Autodesk Inventor part; units mm, degrees
ref_plane "Work Plane1" through (104.775, 0, 0) normal (0, 0, -1) x (1, 0, 0)
ref_plane "YZ Plane" through (0, 0, 0) normal (1, 0, 0) x (0, 1, 0)
ref_plane "XZ Plane" through (0, 0, 0) normal (0, 1, 0) x (-1, 0, 0)
sketch "Sketch1" plane through (0, 0, 0) normal (0, 0, 1) x (1, 0, 0)
  line L0 (20, 0) -> (20, 2)
  line L1 (20, 2) -> (5, 2)
  line L2 (5, 2) -> (4.5706, 2)
  line L3 (0, 3.765) -> (0, 1.4434)
  line L4 (0, 1.4434) -> (1.78, 1.4434)
  line L5 (1.78, 1.4434) -> (2.6133, 0)
  line L6 (2.6133, 0) -> (20, 0)
  line L7 (0, 3.765) -> (0.715, 3.765)
  line L8 (0.715, 3.765) -> (2.48, 2)
  line L9 (4.5706, 2) -> (2.48, 2)
  line L10 (5, 2) -> (2.48, 2) construction
  line L11 (2.48, 2) -> (2.48, 2)
  line L12 (-4, 0) -> (24, 0)
  line L13 (0, -0.753) -> (0, 4.518)
  dimension "d0" = 20
  dimension "d1" = 15
  dimension "d2" = 1.78
  dimension "d3" = 4
  dimension "d6" = 2.48
  dimension "d7" = 45
  dimension "d8" = 2.8868
  dimension "d9" = 60
  dimension "d10" = 7.53
  dimension "d11" = 4
  dimension "d12" = 0.4294
revolve "Body" add sketch "Sketch1" angle 360 about axis through (2.6133, 0, 0) along (1, 0, 0) contours L6 L5 L4 L3 L7 L8 L9 L2 L1 L0
sketch "Sketch2" plane through (0, 0, 0) normal (-1, 0, 0) x (0, 0, 1)
  circle A0 centre (0, 0) radius 1.4434
  line L0 (0, -5.271) -> (0, 5.271)
  line L1 (-5.271, 0) -> (5.271, 0)
  line L2 (1.4434, 0) -> (0.7217, -1.25)
  line L3 (0.7217, -1.25) -> (-0.7217, -1.25)
  line L4 (-0.7217, -1.25) -> (-1.4434, 0)
  line L5 (-1.4434, 0) -> (-0.7217, 1.25)
  line L6 (-0.7217, 1.25) -> (0.7217, 1.25)
  line L7 (0.7217, 1.25) -> (1.4434, 0)
  point P0 (0, 1.4434)
extrude "Slot" add sketch "Sketch2" against normal up to next contours L7 A0 | A0 L2 | L6 L0 A0 | A0 L0 L3 | L0 L6 A0 | A0 L3 L0 | L4 A0 | A0 L5
thread "Thread"
chamfer "Chamfer1" distance 0.4294 distance2 0.4294 1 edges at (20, -2, 0) measured on face at (20, -0.7974, -0.7684)
ref_plane "Work Plane1" through (104.775, 0, 0) normal (0, 0, -1) x (1, 0, 0)
equation "\"d0\" = NLG"
equation "\"d1\" = GEL"
equation "\"d2\" = INTI"
equation "\"d3\" = GD"
equation "\"d6\" = KOH"
equation "\"d7\" = 0.5 * SEWI"
equation "\"d8\" = 1.1547 * SW"
equation "\"d10\" = KOD"
equation "\"d11\" = BDM"
equation "\"d12\" = GAL"
equation "\"d15\" = GEL"
equation "\"d17\" = -0.5 * SPD + 0.5 * GD"
equation "\"d18\" = GUL"
equation "\"NLG\" = 20"
equation "\"INTI\" = 1.78"
equation "\"GEL\" = 15"
equation "\"GAL\" = 0.61345 * PTC"
equation "\"KOH\" = 2.48"
equation "\"KOD\" = 7.53"
equation "\"GUL\" = 0.61345 * PTC"
equation "\"SPD\" = NND - 1.2269 * PTC"
equation "\"BDM\" = NND"
equation "\"GD\" = NND"
equation "\"SEWI\" = 90deg"
equation "\"SW\" = 2.5"
equation "\"TOA\" = 30deg"
equation "\"GD1\" = THREADDIA - 1.2269 * PTC"
equation "\"EPV\" = 4.48"
equation "\"THREADDIA\" = 4"
equation "\"PTC\" = 0.7"
equation "\"NND\" = 4"
equation "\"E0\" = 2.89"
equation "\"THREADDESC\" = 1.2345"
properties part number "451233010040020" material "Stainless Steel"
Design review of the part built by this model. Coordinates are the model's own, in mm. A direction names the side the tool comes from. Give positions to 0.01 mm unless a question says otherwise; leave off trailing zeros. Write each loop counter-clockwise with the first axis right and the second up, starting at its lowest first coordinate (ties: lowest second). Pieces come first, ordered by that corner, then holes.
(1) Add section A-A (x = 4.5). Give the boundary of the cut face in (y, z), and give its area (3 significant figures).
Checked values:
outline: circle Ø4 at (0, 0)
area: 12.6 mm2
(2) Tool access review of faces 1 (the face through (20, 0, 0)), 2 (the face through (11, 0, 2)), 3 (the face through (0.933, -0.616, 1.088)): name each direction out of +Z, -Z, +X, -X, +Y, -Y from which nothing blocks a thin tool from reaching the whole face with its end or side.
Checked values:
face 1: +Z, -Z, +X, +Y, -Y
face 2: +X
face 3: -X
(3) Wall thickness on line 1 along X through (y, z) = (2.25, 1.25); line 2 along X through (y, z) = (2.75, 1.25); line 3 along Y through (x, z) = (13, 0.75): over which ranges is each line inside the solid? List them lowest first.
Checked values:
line 1: x = 0 to 1.91
line 2: x = 0 to 1.46
line 3: y = -1.85 to 1.85
(4) Clearance check with flat-ended pins moving along their axes: pin 1 Ø1.5 at (x, z) = (11.5, -2.5) entering from -Y; pin 2 Ø1 at (x, z) = (2.5, -3) entering from -Y; pin 3 Ø1 at (x, z) = (8.5, -0.5) entering from -Y; pin 4 Ø1 at (y, z) = (1.5, -3) entering from +X. State where each tip first meets the part, or that it passes through.
Checked values:
pin 1: stops at y = -0.97
pin 2: passes through
pin 3: stops at y = -2
pin 4: stops at x = 1.63
(5) Mouldability with a two-part tool opening along Z and no side actions: class faces 4 (the face through (2.37, -0.46, 2.06)), 5 (the face through (0, 0, 2)), 6 (the face through (1, 1.25, 0)) as +Z half, -Z half, draft (parallel to the pull), parting line (faces both ways), or undercut.
Checked values:
face 4: parting line
face 5: draft
face 6: undercut
